For this review, take the finished solid that the model builds, in its own axes (mm). Round coordinates to 2 decimals unless told otherwise and drop trailing zeros. Write each loop counter-clockwise with the first axis right and the second up, starting at its lowest first coordinate (ties: lowest second). Pieces come first, ordered by that corner, then holes.
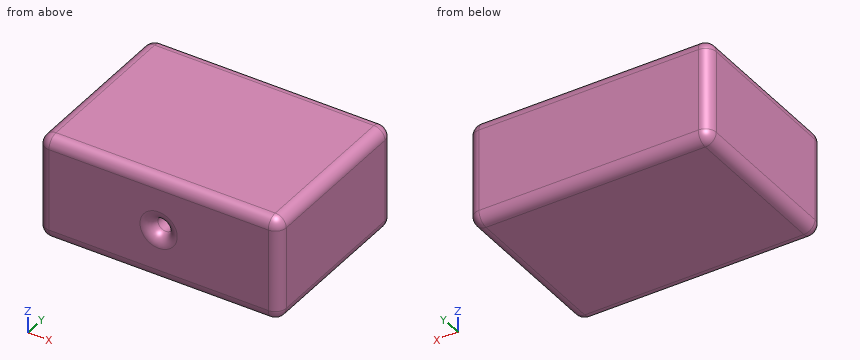
from build123d import *

# Parameters (mm, degrees)
F0_W     = 110.007778
F0_H     = 47.554146
F1_DEPTH = 80
F2_R     = 3.5
F3_DEPTH = 40
F4_R     = 5


with BuildPart() as f1:
    # F0 (on Front) → F1 (new body)
    with BuildSketch(Plane.XZ):
        Rectangle(F0_W, F0_H)
    extrude(amount=F1_DEPTH)

    # F2 (on face) → F3 (cut)
    with BuildSketch(Plane.XZ.offset(80)):
        Circle(F2_R)
    extrude(amount=-F3_DEPTH, mode=Mode.SUBTRACT)

    # F4
    f4_edges = [f1.edges().sort_by_distance(p)[0] for p in [
        (0, -80, 23.777073),
        (-55.003889, -80, 0),
        (0, -80, -23.777073),
        (55.003889, -80, 0),
        (-55.003889, -40, 23.777073),
        (0, 0, 23.777073),
        (55.003889, -40, 23.777073),
        (55.003889, -40, -23.777073),
        (-55.003889, -40, -23.777073),
        (0, 0, -23.777073),
        (55.003889, 0, 0),
        (-55.003889, 0, 0),
        (-3.5, -80, 0),
    ]]
    fillet(f4_edges, radius=F4_R)


solid = f1.part
(1) We need section B-B, the plane x = 0. Give the boundary of the cut face in (y, z), and give its area (3 significant figures).
Geometry check:
outline: (-80, -18.78) arc R5 ccw to (-75, -23.78) - (-5, -23.78) arc R5 ccw to (0, -18.78) - (0, 18.78) arc R5 ccw to (-5, 23.78) - (-75, 23.78) arc R5 ccw to (-80, 18.78) - (-80, 8.5) arc R5 ccw to (-75, 3.5) - (-40, 3.5) - (-40, -3.5) - (-75, -3.5) arc R5 ccw to (-80, -8.5) - close
area: 3,490 mm2
(2) For line 1 along Z through (x, y) = (0, -58); line 2 along Z through (x, y) = (29, -4); line 3 along Y through (x, z) = (-6, -1), list the stretches that pass through material, from the lowest coordinate up.
Geometry check:
line 1: z = -23.78 to -3.5, 3.5 to 23.78
line 2: z = -23.68 to 23.68
line 3: y = -79.38 to 0
(3) We need section A-A, the plane z = 0. Give the boundary of the cut face in (x, y), and give its area (3 significant figures).
Geometry check:
outline: (-55, -75) arc R5 ccw to (-50, -80) - (-8.5, -80) arc R5 ccw to (-3.5, -75) - (-3.5, -40) - (3.5, -40) - (3.5, -75) arc R5 ccw to (8.5, -80) - (50, -80) arc R5 ccw to (55, -75) - (55, -5) arc R5 ccw to (50, 0) - (-50, 0) arc R5 ccw to (-55, -5) - close
area: 8,490 mm2
(4) For pin 1 Ø3.5 at (x, z) = (-1.5, 0.5) entering from -Y; pin 2 Ø8 at (x, z) = (0, 0) entering from -Y, all flat-tipped, find the tip position at first contact; note any pin that passes through.
Geometry check:
pin 1: stops at y = -40
pin 2: stops at y = -77.18
